from build123d import *

# Parameters (mm, degrees)
SKETCH1_R           = 1.25
BOSS_EXTRUDE1_DEPTH = 6.35


with BuildPart() as part:
    # Sketch1 → Boss-Extrude1 (new body)
    with BuildSketch(Plane(origin=(0, 0, 0), x_dir=(1, 0, 0), z_dir=(0, 1, 0))):
        with BuildLine():
            Line((-12.884325045, 57.589892951), (-32.880086413, 58.0016299))
            Line((-32.880086413, 58.0016299), (-30.409664718, 177.976198108))
            Line((-30.409664718, 177.976198108), (264.52781546, 171.903078107))
            Line((264.52781546, 171.903078107), (262.674606435, 81.903078107))
            ThreePointArc((262.674606435, 81.903078107), (245.966301841, 93.936578204), (228.109303454, 104.188415872))
            Line((228.109303454, 104.188415872), (239.565645069, 129.341286502))
            Line((239.565645069, 129.341286502), (207.713903894, 143.848752998))
            Line((207.713903894, 143.848752998), (195.598020496, 117.247831174))
            ThreePointArc((195.598020496, 117.247831174), (165.438476431, 123.896281605), (134.614931972, 125.822183564))
            Line((134.614931972, 125.822183564), (134.614931972, 150.073013143))
            Line((134.614931972, 150.073013143), (99.614931972, 150.073013143))
            Line((99.614931972, 150.073013143), (99.614931972, 122.205605467))
            ThreePointArc((99.614931972, 122.205605467), (64.494604203, 112.00765114), (31.818351454, 95.585160423))
            Line((31.818351454, 95.585160423), (15.189825734, 117.890629233))
            Line((15.189825734, 117.890629233), (-12.870789642, 96.971693679))
            Line((-12.870789642, 96.971693679), (3.847059798, 74.546406222))
            ThreePointArc((3.847059798, 74.546406222), (-4.771312567, 66.317474746), (-12.884325045, 57.589892951))
        make_face()
        with Locations(Location((-20.617652508, 167.77244895, 0), (0, 0, 270))):
            Circle(SKETCH1_R, mode=Mode.SUBTRACT)
        with Locations(Location((254.324066301, 162.111065898, 0), (0, 0, 270))):
            Circle(SKETCH1_R, mode=Mode.SUBTRACT)
        with Locations(Location((-22.676337254, 67.79364211, 0), (0, 0, 270))):
            Circle(SKETCH1_R, mode=Mode.SUBTRACT)
    extrude(amount=BOSS_EXTRUDE1_DEPTH)


solid = part.part
The listing builds one solid part. Answer for the finished solid, in the listing's coordinates (mm). A direction names the side the tool comes from. Round coordinates to 2 decimals unless told otherwise and drop trailing zeros. Order: outer loops, then holes, each group sorted by start corner. A loop starts at its lowest first (then second) coordinate and runs counter-clockwise, first axis right, second up. Notation, with made-up numbers: (77.25, -0.5) -> (123.25, -0.5) arc R23 cw to (123.25, 32.5) -> close; hole circle Ø5 at (44.5, 17.25). An arc over 180 degrees is marked (long way). Write each question's results on one line, items separated by ' | '. Start each with the question number.
Q1. The mould has two halves that part along Z. Classify faces 4 (the cylindrical face through (-4.65, 3.13, -66.44)), 5 (the flat face through (233.76, 3.13, -116.59)), 6 (the flat face through (134.615, 3, -138)), 7 (the flat face through (223.863, 3.131, -136.493)): pulls with the +Z half, pulls with the -Z half, needs draft (parallel to the pull), parting line crosses it, or undercut.
Q2. Straight lines are drawn through the part: probe 1 along X at (y, z) = (5.5, -110.5); probe 2 along X at (y, z) = (1.75, -139.5); probe 3 along Z at (x, y) = (-7.5, 5.5). For each, find the intervals that lie inside material, in ascending order. Write a range as from..to.
Q3. Find section A-A (z = -136). Determine the outline of the cut face in (x, y).
Q4. Find section C-C (y = 4.5). Determine the outline of the cut face in (x, z), then the cut area to 3 significant figures.
Q5. Each of these flat-tipped pins is pushed along its axis until it touches: pin 1 (3 mm diameter, centred on x = 149.5, y = 4, fed in from +Z); pin 2 (1.9 mm diameter, centred on y = 2, z = -143, fed in from +X); pin 3 (1.9 mm diameter, centred on y = 3.5, z = -134, fed in from -X). Where does it stop, or does it pass through?
Q6. Which of the six approach directions +Z, -Z, +X, -X, +Y, -Y give full straight-line access (tool end or side, diameter ignored) to faces 1 (the cylindrical face through (64.972, 3.131, -112.194)), 2 (the flat face through (85, 0, -145)), 3 (the flat face through (-4.63, 3.13, -85.92))?
Q7. Find section D-D (z = -87). Determine the outline of the cut face in (x, y), then the cut area to 3 significant figures.
Q8. Find section B-B (x = -8). Determine the outline of the cut face in (y, z), then the cut area to 3 significant figures.
Worked answers:
1) face 4: pulls with the +Z half | face 5: undercut | face 6: needs draft | face 7: undercut
2) probe 1: x = -31.8..5.28, 20.7..60.77, 230.98..263.26 | probe 2: x = -31.2..99.61, 134.61..205.73, 217.26..263.86 | probe 3: z = -177.5..-100.98, -89.77..-63.5
3) outline: (-31.27, 0) -> (99.61, 0) -> (99.61, 6.35) -> (-31.27, 6.35) -> close; (134.61, 0) -> (204.14, 0) -> (204.14, 6.35) -> (134.61, 6.35) -> close; (224.95, 0) -> (263.79, 0) -> (263.79, 6.35) -> (224.95, 6.35) -> close
4) outline: (-32.88, -58) -> (-30.41, -177.98) -> (264.53, -171.9) -> (262.67, -81.9) arc R200 cw to (228.11, -104.19) -> (239.57, -129.34) -> (207.71, -143.85) -> (195.6, -117.25) arc R200 cw to (134.61, -125.82) -> (134.61, -150.07) -> (99.61, -150.07) -> (99.61, -122.21) arc R200 cw to (31.82, -95.59) -> (15.19, -117.89) -> (-12.87, -96.97) -> (3.85, -74.55) arc R200 cw to (-12.88, -57.59) -> close; hole circle Ø2.5 at (-22.68, -67.79); hole circle Ø2.5 at (-20.62, -167.77); hole circle Ø2.5 at (254.32, -162.11) | area: 17,900 mm2
5) pin 1: stops at z = -125.39 | pin 2: stops at x = 263.95 | pin 3: stops at x = -31.33
6) face 1: +Z, +Y, -Y | face 2: +Z, -Z, +X, -X, -Y | face 3: +Y, -Y
7) outline: (-32.28, 0) -> (-5.44, 0) -> (-5.44, 6.35) -> (-32.28, 6.35) -> close; (256.04, 0) -> (262.78, 0) -> (262.78, 6.35) -> (256.04, 6.35) -> close | area: 213 mm2
8) outline: (0, -177.51) -> (6.35, -177.51) -> (6.35, -100.6) -> (0, -100.6) -> close; (0, -90.44) -> (6.35, -90.44) -> (6.35, -62.97) -> (0, -62.97) -> close | area: 663 mm2
